Design review of the part built by this model. Coordinates are the model's own, in mm. Coordinates: 2 decimals unless noted, no trailing zeros. Loops run counter-clockwise (first coordinate to the right, second up) from the corner with the lowest first, then second, coordinate; pieces in that order, holes last.
Q1. Add section A-A on z = 6. Give the boundary of the cut face in (x, y), and give its area (3 significant figures).
Q2. For P1, Ø1, axis at y = 5, z = 45.5, coming from the +X side; P2, Ø5, axis at x = 24.5, z = 10, coming from the -Y side; P3, Ø1.5, axis at y = -4.5, z = 19, coming from the +X side, all flat-tipped, find the tip position at first contact; note any pin that passes through.
Q3. Add section B-B on y = -35. Give the boundary of the cut face in (x, z).
Q4. Wall thickness on probe 1 along Y at (x, z) = (14.5, -31); probe 2 along Z at (x, y) = (-18.5, 36); probe 3 along Z at (x, y) = (-20, 15.5): over which ranges is each line inside the solid? List them lowest first.
Q5. Add section C-C on z = -13. Give the boundary of the cut face in (x, y), and give its area (3 significant figures).
```python
from build123d import *

# Parameters (mm, degrees)
BOX_W             = 10
BOX_H             = 2.5
BOX_DEPTH         = 10
BOX_ROLL_ANGLE    = 45
BOX001_W          = 10
BOX001_H          = 2.5
BOX001_DEPTH      = 10
BOX001_ROLL_ANGLE = -45
TORUS_R           = 5
TORUS_PITCH_ANGLE = 90


with BuildPart() as obj1:
    # Box → Box (new body)
    with BuildSketch(Plane.XY):
        with Locations((5, 1.25)):
            Rectangle(BOX_W, BOX_H)
    extrude(amount=BOX_DEPTH)


with BuildPart() as obj1_1:
    # Box roll: moved
    add(obj1.part.rotate(Axis((0, 0, 0), (1, 0, 0)), BOX_ROLL_ANGLE))


with BuildPart() as obj1_2:
    # Box placement: moved
    add(obj1_1.part.moved(Location((42, -17, -25))))


with BuildPart() as obj2:
    # Box001 → Box001 (new body)
    with BuildSketch(Plane.XY):
        with Locations((5, 1.25)):
            Rectangle(BOX001_W, BOX001_H)
    extrude(amount=BOX001_DEPTH)


with BuildPart() as obj2_1:
    # Box001 roll: moved
    add(obj2.part.rotate(Axis((0, 0, 0), (1, 0, 0)), BOX001_ROLL_ANGLE))


with BuildPart() as obj2_2:
    # Box001 placement: moved
    add(obj2_1.part.moved(Location((42, -24, -23))))


with BuildPart() as obj3:
    # Torus → Torus (revolve)
    with BuildSketch(Plane.XZ):
        with Locations((20, 0)):
            Circle(TORUS_R)
    revolve(axis=Axis((0, 0, 0), (0, 0, 1)))


with BuildPart() as obj3_1:
    # Torus pitch: moved
    add(obj3.part.rotate(Axis((0, 0, 0), (0, 1, 0)), TORUS_PITCH_ANGLE))


with BuildPart() as obj3_2:
    # Torus placement: moved
    add(obj3_1.part.moved(Location((0, 0, 50))))


with BuildPart() as obj4:
    # Sphere001 → Sphere001 (revolve)
    with BuildSketch(Plane(origin=(40, -20, -20), x_dir=(1, 0, 0), z_dir=(0, -1, 0))):
        with BuildLine():
            ThreePointArc((0, -10), (10, 0), (0, 10))
            Line((0, 10), (0, -10))
        make_face()
    revolve(axis=Axis((40, -20, -20), (0, 0, 1)))


with BuildPart() as cut001:
    # Sphere → Sphere (revolve)
    with BuildSketch(Plane.XZ):
        with BuildLine():
            ThreePointArc((0, -50), (50, 0), (0, 50))
            Line((0, 50), (0, -50))
        make_face()
    revolve(axis=Axis((0, 0, 0), (0, 0, 1)))

    # Fusion: union obj4
    add(obj4.part)

    # Fusion001: union obj3
    add(obj3_2.part)

    # Cut: cut obj2
    add(obj2_2.part, mode=Mode.SUBTRACT)

    # Cut001: cut obj1
    add(obj1_2.part, mode=Mode.SUBTRACT)


solid = cut001.part
```
Entries:
1. outline: circle Ø99.28 at (0, 0)
1. area: 7,740 mm2
2. P1: stops at x = 21.22
2. P2: stops at y = -43.88
2. P3: stops at x = 46.34
3. outline: circle Ø71.41 at (0, 0)
4. probe 1: y = -36.45 to 36.45
4. probe 2: z = -29.36 to 29.36
4. probe 3: z = -43.12 to 43.12
5. outline: (39.93, -27.14) arc R7.14 ccw to (45.67, -15.66) arc R48.28 ccw (long way) to start
5. area: 7,360 mm2
